Verification items for the finished model (mm, model axes). A direction names the side the tool comes from. Round coordinates to 2 decimals unless told otherwise and drop trailing zeros. Write each loop counter-clockwise with the first axis right and the second up, starting at its lowest first coordinate (ties: lowest second). Pieces come first, ordered by that corner, then holes. Notation, with made-up numbers: M -18.75,-1 L 2.25,-1 A27 cw 2.25,25 Z; hole C 55.5,72 d7. An arc over 180 degrees is marked long. Write each question's results on one line, items separated by ' | '.
from build123d import *

# Parameters (mm, degrees)
SKETCH1_W           = 4
SKETCH1_H           = 3.5
SKETCH2_R           = 2
BOSS_EXTRUDE1_DEPTH = 12
CUT_EXTRUDE1_DEPTH  = 2
CHAMFER1_SIZE       = 0.39
FILLET1_R           = 0.2


with BuildPart() as part:
    # Sketch1 → Revolve1 (revolve)
    with BuildSketch(Plane(origin=(0, 0, 0), x_dir=(-1, 0, 0), z_dir=(0, 0, -1))):
        with Locations((-2, 1.75)):
            Rectangle(SKETCH1_W, SKETCH1_H)
    revolve(axis=Axis((4, 0, 0), (-1, 0, 0)))

    # Sketch2 → Boss-Extrude1 (add)
    with BuildSketch(Plane(origin=(4, 0, 0), x_dir=(0, 0, -1), z_dir=(1, 0, 0))):
        Circle(SKETCH2_R)
    extrude(amount=BOSS_EXTRUDE1_DEPTH)

    # Sketch3 → Cut-Extrude1 (cut)
    with BuildSketch(Plane.ZY):
        Polygon((1.5355, -0.886521338), (1.5355, 0.886521338), (0, 1.773042677), (-1.5355, 0.886521338), (-1.5355, -0.886521338), (0, -1.773042677), align=None)
    extrude(amount=-CUT_EXTRUDE1_DEPTH, mode=Mode.SUBTRACT)

    # Sketch4 → Cut-Revolve1 (revolve, cut)
    with BuildSketch(Plane.XY):
        Polygon((2, 1.5355), (2, 0), (2.886521338, 0), align=None)
    revolve(axis=Axis((2, 0, 0), (1, 0, 0)), mode=Mode.SUBTRACT)

    # Chamfer1
    chamfer1_edges = [part.edges().sort_by_distance(p)[0] for p in [
        (0, -3.5, 0),
        (16, 0, 2),
    ]]
    chamfer(chamfer1_edges, length=CHAMFER1_SIZE)

    # Fillet1
    fillet1_edges = [part.edges().sort_by_distance(p)[0] for p in [
        (4, 0, 2),
    ]]
    fillet(fillet1_edges, radius=FILLET1_R)


solid = part.part
1) Depth check by flat-ended pin: P1, Ø2, axis at x = 9.5, y = 2.5, coming from the +Z side; P2, Ø0.6, axis at y = 0.5, z = 1, coming from the -X side; P3, Ø1, axis at y = 2.5, z = -2.5, coming from the +X side. Enter the tip coordinate at first touch or a pass-through.
Calculated:
P1: stops at z = 1.32 | P2: stops at x = 2.07 | P3: stops at x = 4
2) Sectioned sample at A-A, the plane x = 12. Record the cut outline in (y, z).
Calculated:
outline: C 0,0 d4
3) Material ranges on line 1 (Y direction, x = 1.75, z = 1.25); line 2 (X direction, y = 3, z = -0.5); line 3 (Y direction, x = 2.75, z = 0), recorded low to high. Write a range as [from, to].
Calculated:
line 1: y = [-3.27, -1.05], [1.05, 3.27] | line 2: x = [0, 4] | line 3: y = [-3.5, -0.24], [0.24, 3.5]
4) Access from +Z, -Z, +X, -X, +Y, -Y to the whole of each face (thin tool, end or side, straight path). Record for faces 4 (the cylindrical face through (10, -2, 0)), 5 (the flat face through (0.986, 1.336, -0.757)), 6 (the flat face through (16, 0, 0)).
Calculated:
face 4: +X | face 5: -X | face 6: +Z, -Z, +X, +Y, -Y
5) Draft check along Y on faces 1 (the flat face through (0.986, -1.336, 0.757)), 2 (the flat face through (4, 2, 2)), 3 (the cylindrical face through (2.17, 3.233, 1.341)). Enter one of: pulls with the +Y half, pulls with the -Y half, needs draft (parallel to the pull), parting line crosses it, or undercut.
Calculated:
face 1: undercut | face 2: needs draft | face 3: parting line crosses it
